Geometry: final body of the model. Coordinates: model frame, mm. A direction names the side the tool comes from. Give positions to 0.01 mm unless a question says otherwise; leave off trailing zeros. Write each loop counter-clockwise with the first axis right and the second up, starting at its lowest first coordinate (ties: lowest second). Pieces come first, ordered by that corner, then holes.
```python
from build123d import *

# Parameters (mm, degrees)
PAD003_DEPTH    = 3
PAD002_DEPTH    = 3
PAD001_DEPTH    = 3
SKETCH_W        = 20
SKETCH_H        = 20
PAD_DEPTH       = 10
SKETCH001_R     = 6
POCKET_DEPTH    = 18
SKETCH003_R     = 6
POCKET001_DEPTH = 18
SKETCH004_R     = 6
POCKET002_DEPTH = 18
SKETCH005_R     = 3.5
POCKET003_DEPTH = 5
SKETCH006_R     = 3.5
POCKET004_DEPTH = 5
SKETCH007_R     = 3.5
POCKET005_DEPTH = 5
SKETCH011_R     = 0.5
PAD004_DEPTH    = 2
SKETCH012_R     = 0.5
PAD005_DEPTH    = 2
SKETCH013_R     = 0.5
PAD006_DEPTH    = 2


with BuildPart() as pad003:
    # Sketch010 → Pad003 (new body, symmetric)
    with BuildSketch(Plane.YZ):
        Polygon((5, -10), (10, -10), (10, -5), align=None)
    extrude(amount=PAD003_DEPTH, both=True)


with BuildPart() as pad002:
    # Sketch009 → Pad002 (new body, symmetric)
    with BuildSketch(Plane.XZ):
        Polygon((5, -10), (10, -10), (10, -5), align=None)
    extrude(amount=PAD002_DEPTH, both=True)


with BuildPart() as pad001:
    # Sketch008 → Pad001 (new body, symmetric)
    with BuildSketch(Plane.XY):
        Polygon((10, 5), (5, 10), (10, 10), align=None)
    extrude(amount=PAD001_DEPTH, both=True)


with BuildPart() as pad006:
    # Sketch → Pad (new body, symmetric)
    with BuildSketch(Plane.XZ):
        Rectangle(SKETCH_W, SKETCH_H)
    extrude(amount=PAD_DEPTH, both=True)

    # Sketch001 → Pocket (cut)
    with BuildSketch(Plane.XZ.offset(10)):
        Circle(SKETCH001_R)
    extrude(amount=-POCKET_DEPTH, mode=Mode.SUBTRACT)

    # Sketch003 → Pocket001 (cut)
    with BuildSketch(Plane(origin=(0, 0, 10), x_dir=(-1, 0, 0), z_dir=(0, 0, 1))):
        Circle(SKETCH003_R)
    extrude(amount=-POCKET001_DEPTH, mode=Mode.SUBTRACT)

    # Sketch004 → Pocket002 (cut)
    with BuildSketch(Plane(origin=(-10, 0, 0), x_dir=(0, 0, -1), z_dir=(-1, 0, 0))):
        Circle(SKETCH004_R)
    extrude(amount=-POCKET002_DEPTH, mode=Mode.SUBTRACT)

    # Sketch005 → Pocket003 (cut)
    with BuildSketch(Plane(origin=(0, 0, -10), x_dir=(1, 0, 0), z_dir=(0, 0, -1))):
        Circle(SKETCH005_R)
    extrude(amount=-POCKET003_DEPTH, mode=Mode.SUBTRACT)

    # Sketch006 → Pocket004 (cut)
    with BuildSketch(Plane(origin=(0, 10, 0), x_dir=(1, 0, 0), z_dir=(0, 1, 0))):
        Circle(SKETCH006_R)
    extrude(amount=-POCKET004_DEPTH, mode=Mode.SUBTRACT)

    # Sketch007 → Pocket005 (cut)
    with BuildSketch(Plane(origin=(10, 0, 0), x_dir=(0, 0, 1), z_dir=(1, 0, 0))):
        Circle(SKETCH007_R)
    extrude(amount=-POCKET005_DEPTH, mode=Mode.SUBTRACT)

    # Cut: cut Pad001
    add(pad001.part, mode=Mode.SUBTRACT)

    # Cut001: cut Pad002
    add(pad002.part, mode=Mode.SUBTRACT)

    # Cut002: cut Pad003
    add(pad003.part, mode=Mode.SUBTRACT)

    # Sketch011 → Pad004 (new body)
    with BuildSketch(Plane.YZ.offset(10)):
        with Locations((-5.5, 8.5)):
            Circle(SKETCH011_R)
        with Locations((5.5, 8.5)):
            Circle(SKETCH011_R)
        with Locations((-5.5, -8.5)):
            Circle(SKETCH011_R)
        with Locations((5.5, -8.5)):
            Circle(SKETCH011_R)
    extrude(amount=PAD004_DEPTH)

    # Sketch012 → Pad005 (new body)
    with BuildSketch(Plane(origin=(0, 10, 0), x_dir=(-1, 0, 0), z_dir=(0, 1, 0))):
        with Locations((-5.5, 8.5)):
            Circle(SKETCH012_R)
        with Locations((5.5, 8.5)):
            Circle(SKETCH012_R)
        with Locations((5.5, -8.5)):
            Circle(SKETCH012_R)
        with Locations((-5.5, -8.5)):
            Circle(SKETCH012_R)
    extrude(amount=PAD005_DEPTH)

    # Sketch013 → Pad006 (new body)
    with BuildSketch(Plane(origin=(0, 0, -10), x_dir=(1, 0, 0), z_dir=(0, 0, -1))):
        with Locations((-5.5, 8.5)):
            Circle(SKETCH013_R)
        with Locations((5.5, 8.5)):
            Circle(SKETCH013_R)
        with Locations((-5.5, -8.5)):
            Circle(SKETCH013_R)
        with Locations((5.5, -8.5)):
            Circle(SKETCH013_R)
    extrude(amount=PAD006_DEPTH)


solid = pad006.part
```
Item 1: Section B-B, the plane y = 8.5. Return the cut outline in (x, z), plus the area to 3 significant figures.
Found:
outline: (-10, -10) - (-6, -10) - (-6, -12) - (-5, -12) - (-5, -10) - (-3, -10) - (-3, -6.5) - (3, -6.5) - (3, -10) - (5, -10) - (5, -12) - (6, -12) - (6, -10) - (10, -10) - (10, -3) - (6.5, -3) - (6.5, 3) - (10, 3) - (10, 10) - (-10, 10) - close; hole circle Ø7 at (0, 0)
area: 324 mm2
Item 2: Reachability of faces 4 (the face through (5.608, 10.986, -8.988)), 5 (the face through (0, 8, -7)), 6 (the face through (10.986, 5.392, 8.012)), 7 (the face through (5.392, 8.988, -10.986)) from +Z, -Z, +X, -X, +Y, -Y: full face, straight path, thin tool, end or side. Return the list, or none.
Found:
face 4: +Y
face 5: -Z, +Y
face 6: +X
face 7: -Z
Item 3: Pull-direction query (Z, two-part tool) for faces 1 (the face through (3, 8, -3)), 2 (the face through (4, -5, 10)), 3 (the face through (5.392, -8.012, -10.986)); classes: +Z half, -Z half, draft (parallel to the pull), parting line (faces both ways), or undercut.
Found:
face 1: undercut
face 2: +Z half
face 3: draft
Item 4: Pin query (flat end, axial travel): pin 1 Ø10 at (x, z) = (4.5, 2) entering from +Y; pin 2 Ø10 at (y, z) = (-1.5, 0) entering from +X; pin 3 Ø6 at (x, y) = (6, -5) entering from -Z. Return the tip coordinate at first contact, or that it passes through.
Found:
pin 1: stops at y = 10
pin 2: stops at x = 10
pin 3: stops at z = -10
Item 5: Section A-A, the plane z = 0. Return the cut outline in (x, y), plus the area to 3 significant figures.
Found:
outline: (-10, -10) - (-6, -10) - (-6, -6) - (-10, -6) - close; (-10, 6) - (-6, 6) - (-6, 8) - (-3.5, 8) - (-3.5, 10) - (-10, 10) - close; (3.5, 8) - (6, 8) - (6, 6) - (8, 6) - (8, 3.5) - (10, 3.5) - (10, 5) - (5, 10) - (3.5, 10) - close; (6, -10) - (10, -10) - (10, -3.5) - (8, -3.5) - (8, -6) - (6, -6) - close
area: 71.5 mm2
Item 6: Section C-C, the plane x = 0. Return the cut outline in (y, z).
Found:
outline: (-10, -10) - (-3.5, -10) - (-3.5, -8) - (-6, -8) - (-6, -6) - (-10, -6) - close; (-10, 6) - (-6, 6) - (-6, 10) - (-10, 10) - close; (3.5, -10) - (5, -10) - (10, -5) - (10, -3.5) - (8, -3.5) - (8, -6) - (6, -6) - (6, -8) - (3.5, -8) - close; (6, 6) - (8, 6) - (8, 3.5) - (10, 3.5) - (10, 10) - (6, 10) - close
Item 7: Line query: L1, parallel to Y at x = -7.6, z = 0; L2, parallel to Z at x = 8.25, y = 8.75; L3, parallel to X at y = -4.25, z = 6.25. Output: solid intervals per line, ascending.
Found:
L1: y = -10 to -6, 6 to 10
L2: z = -10 to -3, 3 to 10
L3: x = -10 to -4.24, 4.24 to 10
